For this review, use the dimensioned drawing (mm, ordinates from the lowest corner) and the shaded views. Coordinates: 2 decimals unless noted, no trailing zeros. Order: outer loops, then holes, each group sorted by start corner. A loop starts at its lowest first (then second) coordinate and runs counter-clockwise, first axis right, second up. Notation, with made-up numbers: M -16,-29.75 L -2,-29.75 A11 ccw -2,-13.75 Z; hole C 45,87.25 d11. An arc over 180 degrees is marked long. One line per item, written item: value.
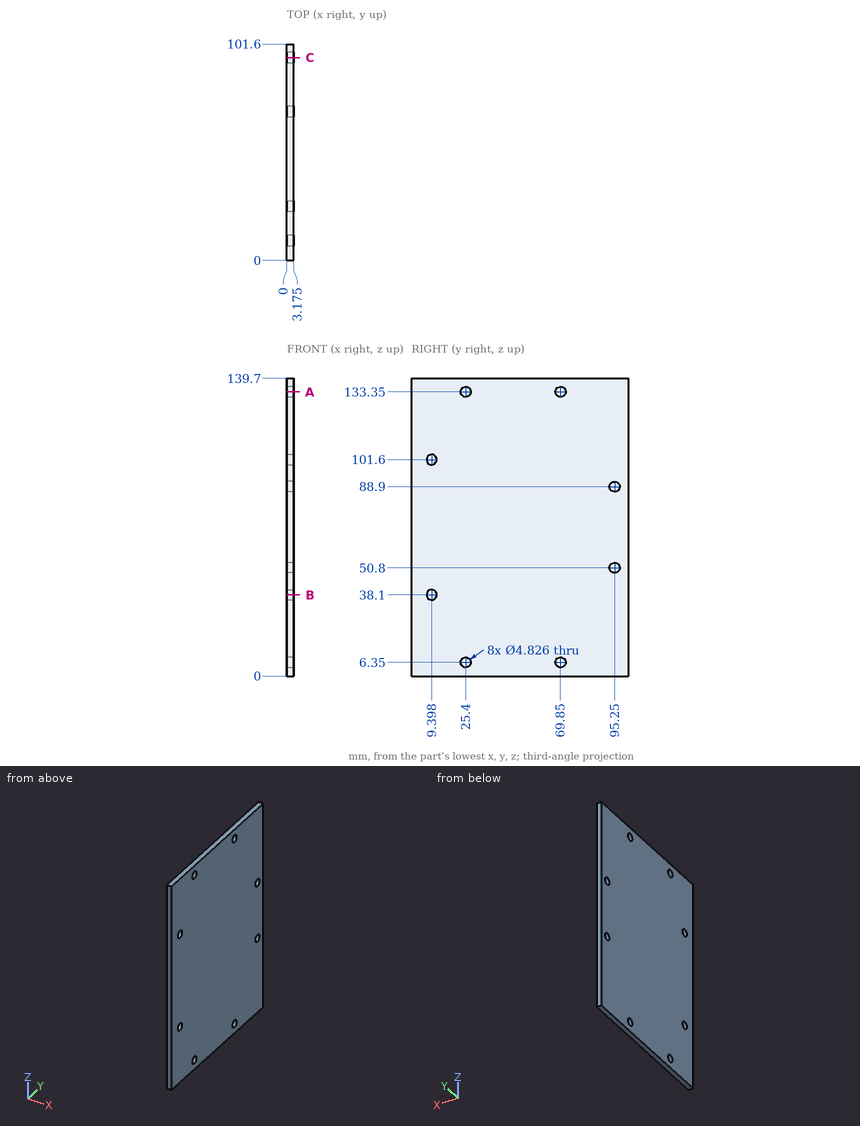
(1) We need section C-C, the plane y = 95.25. State the section outline as (x, z) points (3 decimals), plus the area to 3 significant figures.
Geometry results:
outline: M 0,0 L 3.175,0 L 3.175,48.387 L 0,48.387 Z; M 0,53.213 L 3.175,53.213 L 3.175,86.487 L 0,86.487 Z; M 0,91.313 L 3.175,91.313 L 3.175,139.7 L 0,139.7 Z
area: 413 mm2
(2) We need section B-B, the plane z = 38.1. State the section outline as (x, y) points (3 decimals).
Geometry results:
outline: M 0,0 L 3.175,0 L 3.175,6.985 L 0,6.985 Z; M 0,11.811 L 3.175,11.811 L 3.175,101.6 L 0,101.6 Z
(3) For L1, parallel to Z at x = 2.35, y = 95.25; L2, parallel to Y at x = 0.7, z = 88.9; L3, parallel to Y at x = 3.05, z = 39, list the stretches that pass through material, from the lowest coordinate up.
Geometry results:
L1: z = 0 to 48.39, 53.21 to 86.49, 91.31 to 139.7
L2: y = 0 to 92.84, 97.66 to 101.6
L3: y = 0 to 7.16, 11.64 to 101.6
(4) We need section A-A, the plane z = 133.35. State the section outline as (x, y) points (3 decimals), plus the area to 3 significant figures.
Geometry results:
outline: M 0,0 L 3.175,0 L 3.175,22.987 L 0,22.987 Z; M 0,27.813 L 3.175,27.813 L 3.175,67.437 L 0,67.437 Z; M 0,72.263 L 3.175,72.263 L 3.175,101.6 L 0,101.6 Z
area: 292 mm2
(5) Insertion check: pin 1 Ø3 at (y, z) = (25.4, 133.35) entering from +X; pin 2 Ø5.5 at (y, z) = (95.25, 88.9) entering from -X. Each pin has a flat end and moves straight along its axis. Give the tip position at first contact, or say it passes through.
Geometry results:
pin 1: passes through
pin 2: stops at x = 0
